Can you work these out from the drawing? Everything is in mm from the part's minimum corner. Round coordinates to 2 decimals unless told otherwise and drop trailing zeros. Order: outer loops, then holes, each group sorted by start corner. A loop starts at its lowest first (then second) coordinate and runs counter-clockwise, first axis right, second up. Notation, with made-up numbers: M 34,73.25 L 92,73.25 A11 ccw 92,77.25 Z; hole C 63.5,37 d4. An arc over 180 degrees is marked long. Write each question's results on one line, items separated by ' | '. Start each with the question number.
1. I'm going to push flat-ended pins straight in: pin 1 (2.5 mm diameter, centred on x = 73, z = 64, fed in from +Y); pin 2 (3.5 mm diameter, centred on x = 45, z = 45, fed in from -Y). Where does each tip first touch, or does it pass through?
2. Suppose I cut it at C-C on y = 0.6. Give the number of separate pieces and of enclosed holes in the cut face, and give its area (3 significant figures).
3. Suppose I cut it at B-B on x = 64. Write out the boundary of the cut face in (y, z), and give its area (3 significant figures).
4. Suppose I cut it at D-D on x = 73. Write out the boundary of the cut face in (y, z).
5. Please list where these lines run through material, in increasing order: L1, parallel to Z at x = 16, y = 0.7; L2, parallel to Z at x = 7, y = 1.4; L3, parallel to X at y = 0.8, z = 74.
6. Suppose I cut it at A-A on z = 73. Write out the boundary of the cut face in (x, y), and give its area (3 significant figures).
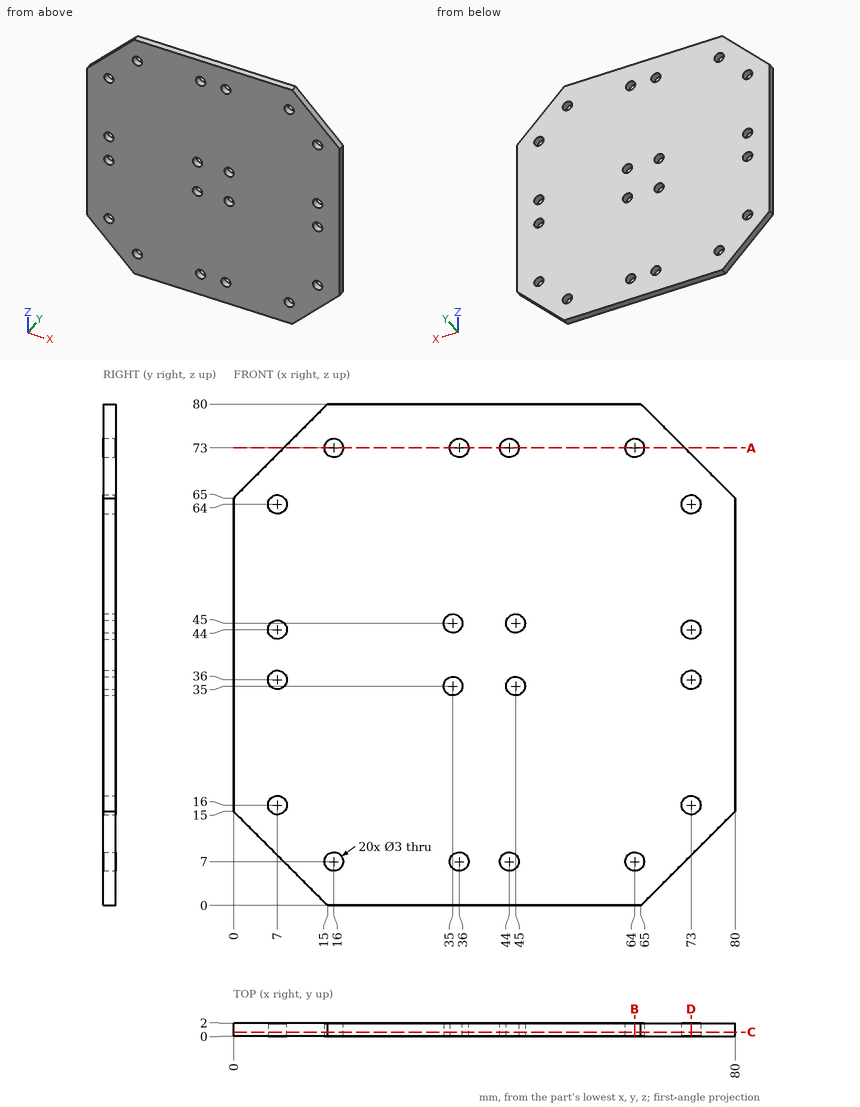
Filled sheet:
1) pin 1: passes through | pin 2: stops at y = 0
2) separate pieces: 1 | enclosed holes: 20 | area: 5,810 mm^2
3) outline: M 0,0 L 2,0 L 2,5.5 L 0,5.5 Z; M 0,8.5 L 2,8.5 L 2,71.5 L 0,71.5 Z; M 0,74.5 L 2,74.5 L 2,80 L 0,80 Z | area: 148 mm^2
4) outline: M 0,8 L 2,8 L 2,14.5 L 0,14.5 Z; M 0,17.5 L 2,17.5 L 2,34.5 L 0,34.5 Z; M 0,37.5 L 2,37.5 L 2,42.5 L 0,42.5 Z; M 0,45.5 L 2,45.5 L 2,62.5 L 0,62.5 Z; M 0,65.5 L 2,65.5 L 2,72 L 0,72 Z
5) L1: z = 0 to 5.5, 8.5 to 71.5, 74.5 to 80 | L2: z = 8 to 14.5, 17.5 to 34.5, 37.5 to 42.5, 45.5 to 62.5, 65.5 to 72 | L3: x = 9 to 14.88, 17.12 to 34.88, 37.12 to 42.88, 45.12 to 62.88, 65.12 to 71
6) outline: M 8,0 L 14.5,0 L 14.5,2 L 8,2 Z; M 17.5,0 L 34.5,0 L 34.5,2 L 17.5,2 Z; M 37.5,0 L 42.5,0 L 42.5,2 L 37.5,2 Z; M 45.5,0 L 62.5,0 L 62.5,2 L 45.5,2 Z; M 65.5,0 L 72,0 L 72,2 L 65.5,2 Z | area: 104 mm^2
